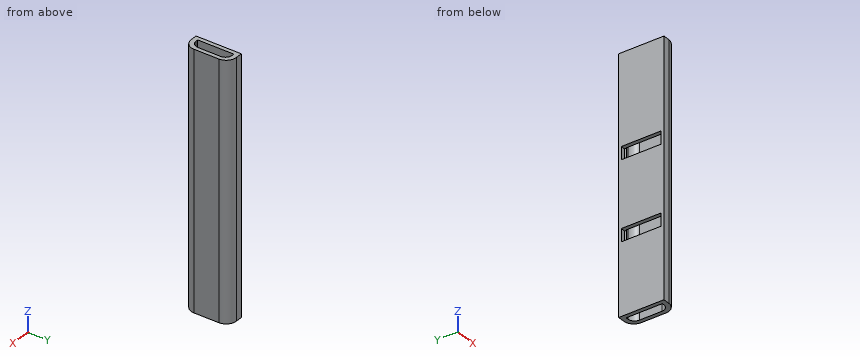
Solid Edge part; units mm, degrees
sketch "Sketch1" plane through (0, 0, 0) normal (0, 0, 1) x (1, 0, 0)
  arc A0 (-2, -16) -> (4, -10) centre (-2, -10) ccw
  line L0 (4, -10) -> (4, 10)
  arc A1 (-2, 16) -> (4, 10) centre (-2, 10) cw
  line L1 (-2, 16) -> (-4, 16)
  line L2 (-4, 16) -> (-4, -16)
  line L3 (-4, -16) -> (-2, -16)
  arc A2 (7.5, -11) -> (-1.5, -20) centre (-1.5, -11) cw
  line L4 (-7.5, -20) -> (-1.5, -20)
  line L5 (-7.5, 20) -> (-7.5, -20)
  line L6 (-1.5, 20) -> (-7.5, 20)
  arc A3 (-1.5, 20) -> (7.5, 11) centre (-1.5, 11) cw
  line L7 (7.5, -11) -> (7.5, 11)
extrude "Protrusion1" add sketch "Sketch1" along normal blind 225
sketch "Sketch2" plane through (-7.5, 0, 112.5) normal (-1, 0, 0) x (0, 0, 1)
  line L0 (21.2, 17.7236) -> (32.5, 17.7236)
  line L1 (32.5, 17.7236) -> (32.5, -17.5764)
  line L2 (32.5, -17.5764) -> (21.2, -17.5764)
  line L3 (21.2, -17.5764) -> (21.2, 17.7236)
  line L4 (-48.8, -17.5764) -> (-37.5, -17.5764)
  line L5 (-37.5, -17.5764) -> (-37.5, 17.7236)
  line L6 (-37.5, 17.7236) -> (-48.8, 17.7236)
  line L7 (-48.8, 17.7236) -> (-48.8, -17.5764)
extrude "VaciadoExtruido_5" cut sketch "Sketch2" against normal blind 4
Source: CAD feature listing. Evaluate the final solid. Frame: model axes, mm. Round coordinates to 2 decimals unless told otherwise and drop trailing zeros. Loops run counter-clockwise (first coordinate to the right, second up) from the corner with the lowest first, then second, coordinate; pieces in that order, holes last. Notation, with made-up numbers: (5, 57.25) - (40, 57.25) arc R13 ccw to (40, 63.25) - close; hole circle Ø6 at (43.5, -39.75). An arc over 180 degrees is marked (long way). Write item = value, one per line. Start each with the question number.
(1) Section query C-C, the plane x = 1. Output: boundary loops of the cut face in (y, z), plus the area to 3 significant figures.
(2) Ray query, line 1 along Z through (x, y) = (-5.5, -5.5); line 2 along X through (y, z) = (5, 54); line 3 along Y through (x, z) = (-1.75, 92.5). Return the intervals inside material, ascending. Write a range as from..to.
(3) Section query D-D, the plane z = 68. Output: boundary loops of the cut face in (x, y), plus the area to 3 significant figures.
(4) Section query A-A, the plane y = 4.5. Output: boundary loops of the cut face in (x, z).
(5) Pin query (flat end, axial travel): pin 1 (1 mm diameter, centred on x = 4, z = 107, fed in from +Y); pin 2 (6 mm diameter, centred on x = 3, z = 55.5, fed in from -Y); pin 3 (0.5 mm diameter, centred on y = 17, z = 71, fed in from -X). Return the tip coordinate at first contact, or that it passes through.
(6) Section query B-B, the plane z = 172. Output: boundary loops of the cut face in (x, y), plus the area to 3 significant figures.
Conclusion:
q1.outline = (-19.65, 0) - (-15.2, 0) - (-15.2, 225) - (-19.65, 225) - close; (15.2, 0) - (19.65, 0) - (19.65, 225) - (15.2, 225) - close
q1.area = 2,000 mm2
q2.line_1 = 0..63.7, 75..133.7, 145..225
q2.line_2 = -7.5..-4, 4..7.5
q2.line_3 = -20..-15.99, 15.99..20
q3.outline = (-7.5, -20) - (-1.5, -20) arc R9 ccw to (7.5, -11) - (7.5, 11) arc R9 ccw to (-1.5, 20) - (-7.5, 20) - (-7.5, 17.72) - (-3.5, 17.72) - (-3.5, 16) - (-2, 16) arc R6 cw to (4, 10) - (4, -10) arc R6 cw to (-2, -16) - (-3.5, -16) - (-3.5, -17.58) - (-7.5, -17.58) - close
q3.area = 199 mm2
q4.outline = (-7.5, 0) - (-4, 0) - (-4, 63.7) - (-7.5, 63.7) - close; (-7.5, 75) - (-4, 75) - (-4, 133.7) - (-7.5, 133.7) - close; (-7.5, 145) - (-4, 145) - (-4, 225) - (-7.5, 225) - close; (4, 0) - (7.5, 0) - (7.5, 225) - (4, 225) - close
q5.pin_1 = 18.48
q5.pin_2 = -19.87
q5.pin_3 = -3.5
q6.outline = (-7.5, -20) - (-1.5, -20) arc R9 ccw to (7.5, -11) - (7.5, 11) arc R9 ccw to (-1.5, 20) - (-7.5, 20) - close; hole (-4, -16) - (-2, -16) arc R6 ccw to (4, -10) - (4, 10) arc R6 ccw to (-2, 16) - (-4, 16) - close
q6.area = 325 mm2
